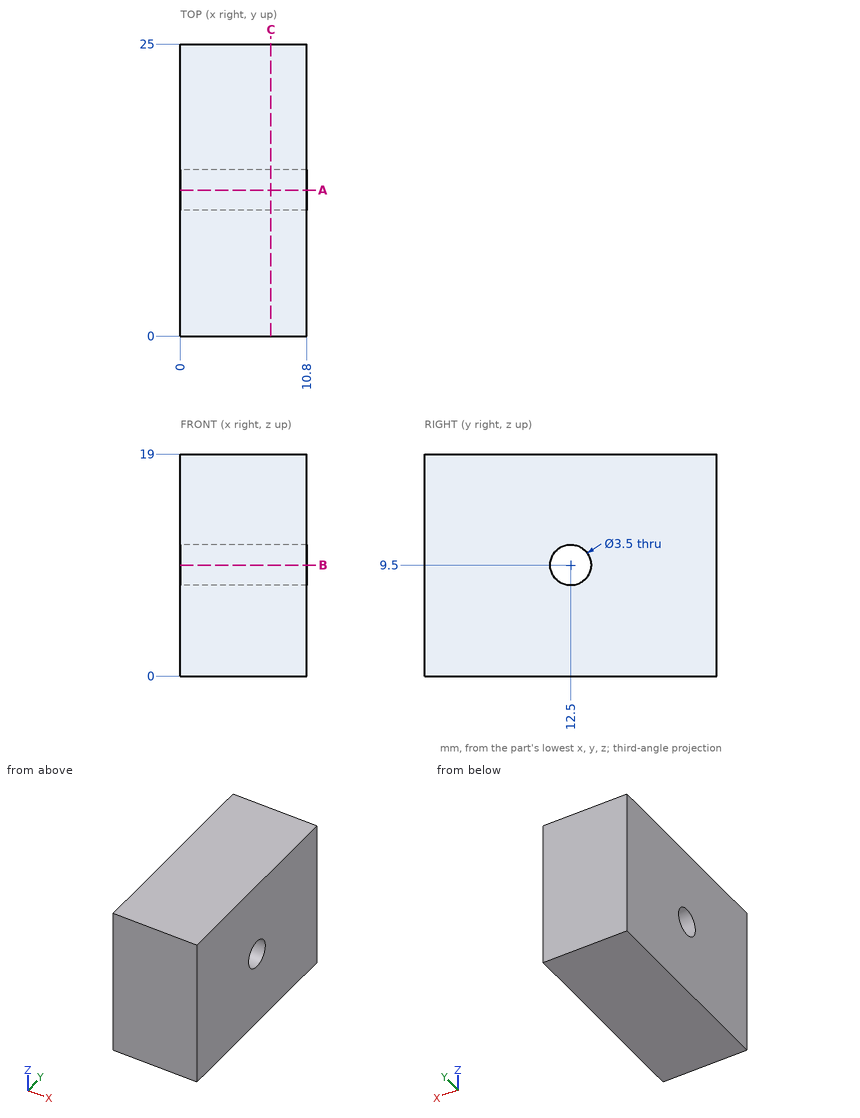
Here's the drawing with two shaded views (mm, measured from the low corner). I have some questions. Round coordinates to 2 decimals unless told otherwise and drop trailing zeros. Loops run counter-clockwise (first coordinate to the right, second up) from the corner with the lowest first, then second, coordinate; pieces in that order, holes last. Notation, with made-up numbers: (87.25, 51) -> (98.25, 51) arc R24 cw to (98.25, 69) -> close; hole circle Ø6 at (81, 49.25). An arc over 180 degrees is marked (long way). Answer as CSV lines item,"result". Start each with the question number.
1. I'm going to push a flat-ended pin straight in: P1, Ø1, axis at x = 8.5, y = 9, coming from the -Z side. Where does the tip first touch, or does it pass through?
2. Imagine slicing it at B-B on z = 9.5. Write out the boundary of the cut face in (x, y), plus the area to 3 significant figures.
3. Imagine slicing it at C-C on x = 7.75. Write out the boundary of the cut face in (y, z), plus the area to 3 significant figures.
4. Imagine slicing it at A-A on y = 12.5. Write out the boundary of the cut face in (x, z), plus the area to 3 significant figures.
5. I need wall thicknesses on probe 1 along Z at (x, y) = (3.25, 12.5); probe 2 along Y at (x, z) = (1.25, 8.5). Which ranges of each line are inside material? Lowest first, please. Write a range as from..to.
Solution:
1,P1,"z = 0"
2,outline,"(0, 0) -> (10.8, 0) -> (10.8, 10.75) -> (0, 10.75) -> close; (0, 14.25) -> (10.8, 14.25) -> (10.8, 25) -> (0, 25) -> close"
2,area,"232 mm²"
3,outline,"(0, 0) -> (25, 0) -> (25, 19) -> (0, 19) -> close; hole circle Ø3.5 at (12.5, 9.5)"
3,area,"465 mm²"
4,outline,"(0, 0) -> (10.8, 0) -> (10.8, 7.75) -> (0, 7.75) -> close; (0, 11.25) -> (10.8, 11.25) -> (10.8, 19) -> (0, 19) -> close"
4,area,"167 mm²"
5,probe 1,"0..7.75, 11.25..19"
5,probe 2,"0..11.06, 13.94..25"
